Autodesk Fusion 360 part; units mm, degrees
sketch "Esquisse1" plane through (0, 0, 0) normal (0, 1, 0) x (1, 0, 0)
  arc A0 (59.719, 39.219) -> (44.719, 54.219) centre (44.719, 39.219) ccw construction
  line L0 (-39.219, -59.719) -> (44.719, -59.719) construction
  line L1 (-54.219, 39.219) -> (-54.219, -44.719) construction
  line L2 (-54.219, 54.219) -> (59.719, -59.719) construction
  line L3 (54.219, -12.5) -> (54.219, 12.5) construction
  arc A1 (44.719, -59.719) -> (59.719, -44.719) centre (44.719, -44.719) ccw construction
  arc A2 (-54.219, -44.719) -> (-39.219, -59.719) centre (-39.219, -44.719) ccw construction
  line L4 (44.719, 54.219) -> (-39.219, 54.219) construction
  line L5 (59.719, -44.719) -> (59.719, 39.219) construction
  arc A3 (-39.219, 54.219) -> (-54.219, 39.219) centre (-39.219, 39.219) ccw construction
  line L6 (-54.519, 39.219) -> (-54.519, -44.719)
  arc A4 (-54.519, -44.719) -> (-39.219, -60.019) centre (-39.219, -44.719) ccw
  line L7 (-39.219, -60.019) -> (44.719, -60.019)
  arc A5 (44.719, -60.019) -> (60.019, -44.719) centre (44.719, -44.719) ccw
  line L8 (60.019, -44.719) -> (60.019, 39.219)
  arc A6 (60.019, 39.219) -> (44.719, 54.519) centre (44.719, 39.219) ccw
  line L9 (44.719, 54.519) -> (-39.219, 54.519)
  arc A7 (-39.219, 54.519) -> (-54.519, 39.219) centre (-39.219, 39.219) ccw
  line L10 (-64.519, 39.219) -> (-64.519, -44.719)
  arc A8 (-64.519, -44.719) -> (-39.219, -70.019) centre (-39.219, -44.719) ccw
  line L11 (-39.219, -70.019) -> (44.719, -70.019)
  arc A9 (44.719, -70.019) -> (70.019, -44.719) centre (44.719, -44.719) ccw
  line L12 (70.019, -44.719) -> (70.019, 39.219)
  arc A10 (70.019, 39.219) -> (44.719, 64.519) centre (44.719, 39.219) ccw
  line L13 (44.719, 64.519) -> (-39.219, 64.519)
  arc A11 (-39.219, 64.519) -> (-64.519, 39.219) centre (-39.219, 39.219) ccw
  line L14 (-39.219, -65.019) -> (44.719, -65.019)
  arc A12 (44.719, -65.019) -> (65.019, -44.719) centre (44.719, -44.719) ccw
  line L15 (65.019, -44.719) -> (65.019, 39.219)
  arc A13 (65.019, 39.219) -> (44.719, 59.519) centre (44.719, 39.219) ccw
  line L16 (44.719, 59.519) -> (-39.219, 59.519)
  arc A14 (-39.219, 59.519) -> (-59.519, 39.219) centre (-39.219, 39.219) ccw
  line L17 (-59.519, 39.219) -> (-59.519, -44.719)
  arc A15 (-59.519, -44.719) -> (-39.219, -65.019) centre (-39.219, -44.719) ccw
  point P0 (54.219, 0)
  point P1 (54.219, 0)
  dimension "d2" = 15
  dimension "d3" = 15
  dimension "d4" = 113.9381
  dimension "d11" = 0.3
  dimension "d12" = 10
  dimension "d13" = 5
extrude "Extrusion1" add sketch "Esquisse1" along normal blind 153 contours L10 A8 L11 A9 L12 A10 L13 A11 | L14 A12 L15 A13 L16 A14 L17 A15
extrude "Extrusion2" cut sketch "Esquisse1" along normal blind 2 contours L14 A12 L15 A13 L16 A14 L17 A15
sketch "Esquisse2" plane through (0, 153, 0) normal (0, 1, 0) x (-1, 0, 0)
  arc A0 (39.219, -54.519) -> (54.519, -39.219) centre (39.219, -39.219) ccw
  line L0 (39.219, -54.519) -> (-44.719, -54.519)
  arc A1 (-60.019, -39.219) -> (-44.719, -54.519) centre (-44.719, -39.219) ccw
  line L1 (-60.019, -39.219) -> (-60.019, 44.719)
  arc A2 (-44.719, 60.019) -> (-60.019, 44.719) centre (-44.719, 44.719) ccw
  line L2 (-44.719, 60.019) -> (39.219, 60.019)
  arc A3 (54.519, 44.719) -> (39.219, 60.019) centre (39.219, 44.719) ccw
  line L3 (54.519, 44.719) -> (54.519, -39.219)
  arc A4 (39.219, -64.519) -> (64.519, -39.219) centre (39.219, -39.219) ccw
  line L4 (64.519, -39.219) -> (64.519, 44.719)
  arc A5 (64.519, 44.719) -> (39.219, 70.019) centre (39.219, 44.719) ccw
  line L5 (39.219, 70.019) -> (-44.719, 70.019)
  arc A6 (-44.719, 70.019) -> (-70.019, 44.719) centre (-44.719, 44.719) ccw
  line L6 (-70.019, 44.719) -> (-70.019, -39.219)
  arc A7 (-70.019, -39.219) -> (-44.719, -64.519) centre (-44.719, -39.219) ccw
  line L7 (-44.719, -64.519) -> (39.219, -64.519)
extrude "Extrusion3" add sketch "Esquisse2" along normal blind 10 contours A0 L0 A1 L1 A2 L2 A3 L3 | A4 L4 A5 L5 A6 L6 A7 L7
fillet "Congé1" radius 2 8 edges at (-54.519, 153, 2.75) (-50.0378, 153, -50.0378) (2.75, 153, -54.519) (55.5378, 153, -50.0378) (60.019, 153, 2.75) (55.5378, 153, 55.5378) (2.75, 153, 60.019) (-50.0378, 153, 55.5378)
fillet "Congé2" radius 1 8 edges at (-64.519, 163, 2.75) (-57.1088, 163, 62.6088) (2.75, 163, 70.019) (62.6088, 163, 62.6088) (70.019, 163, 2.75) (62.6088, 163, -57.1088) (2.75, 163, -64.519) (-57.1088, 163, -57.1088)
sketch "Esquisse3" plane through (-64.519, 0, 0) normal (-1, 0, 0) x (0, 0, 1)
  line L0 (44.719, 162) -> (-39.219, 162)
  line L1 (-39.219, 162) -> (-39.219, 0)
  line L2 (-39.219, 0) -> (44.719, 0)
  line L3 (44.719, 0) -> (44.719, 162)
  line L4 (-10.75, 49) -> (10.75, 49) construction
  line L5 (10.75, 49) -> (10.75, 0) construction
  line L6 (-10.75, 0) -> (-10.75, 49) construction
  circle A0 centre (-7.25, 45.5) radius 1.55
  circle A1 centre (7.25, 45.5) radius 1.55
  line L7 (-7.25, 45.5) -> (7.25, 45.5) construction
  line L8 (2.75, 162) -> (2.75, 132) construction
  line L9 (-17.25, 132) -> (22.75, 132) construction
  circle A2 centre (22.75, 132) radius 5.1
  circle A3 centre (-17.25, 132) radius 5.1
  line L10 (2.75, 132) -> (2.75, 97.36) construction
  circle A4 centre (2.75, 97.36) radius 5.1
  point P0 (2.75, 132)
  dimension "d24" = 49
  dimension "d25" = 21.5
  dimension "d26" = 3.1
  dimension "d27" = 3.1
  dimension "d28" = 14.5
  dimension "d29" = 3.5
  dimension "d30" = 3.5
  dimension "d31" = 30
  dimension "d32" = 40
  dimension "d33" = 34.64
  dimension "d34" = 10.2
  dimension "d35" = 10.2
  dimension "d36" = 10.2
extrude "Extrusion4" cut sketch "Esquisse3" against normal blind 2000 contours A0
extrude "Extrusion5" cut sketch "Esquisse3" against normal blind 2000 contours A1 | A2 | A3 | A4
scale "Echelle2" factor 1.075 about (44.719, 163, -63.519) bodies 1
equation "d4 = ( 430 mm - d2 * ( 2 * 3.141592 - 8 ) ) / 4"
equation "d33 = 0.866 * d32"
The model under review builds one solid part; all positions refer to its coordinate system, in mm. A direction names the side the tool comes from. Round coordinates to 2 decimals unless told otherwise and drop trailing zeros. Write each loop counter-clockwise with the first axis right and the second up, starting at its lowest first coordinate (ties: lowest second). Pieces come first, ordered by that corner, then holes. Notation, with made-up numbers: (15.25, 44) - (20.25, 44) arc R22 cw to (20.25, 62) - close; hole circle Ø5 at (19, 7.5). An arc over 180 degrees is marked (long way). One line per item, written item: value. Start each with the question number.
1. The part is to be moulded in two halves that separate along Y. For faces 1 (the face through (-67, 87, 7)), 2 (the face through (0, 152.25, 9)), 3 (the face through (-64.956, 73.631, -56.415)), say which applies: released by +Y, released by -Y, zero draft, split by the parting line, or undercut.
2. Consider section B-B on z = 7. State how many separate pieces and enclosed holes the cut face has, and give its area (3 significant figures).
3. Consider section C-C on x = 26.5. Write out the cut boundary in (y, z) (3 decimals), and give its area (3 significant figures).
4. Clearance check with flat-ended pins moving along their axes: P1, Ø10, axis at y = 29, z = -45, coming from the +X side; P2, Ø10, axis at x = -22, z = 9, coming from the -Y side. State where each tip first meets the part, or that it passes through.
5. Consider section A-A on y = 112.5. Write out the cut boundary in (x, z) (1 decimal), and give its area (3 significant figures).
6. To check wall thickness, follow L1, parallel to X at y = 136, z = -36; L2, parallel to Z at x = 16, y = 59.5; L3, parallel to Z at x = -21.5, y = 150.5. State the ranges of each line that lie inside material, in increasing order. Write a range as from..to.
7. Machinability: for faces 4 (the face through (-67.41, 135.11, 28.51)), 5 (the face through (59.979, -11.165, -52.996)), which of the approach directions +Z, -Z, +X, -X, +Y, -Y give a long, thin tool a straight path to every point of the face, cutting with its end or side? Answer none if there is none.
Checks:
1. face 1: undercut
1. face 2: released by -Y
1. face 3: zero draft
2. separate pieces: 3
2. enclosed holes: 0
2. area: 4,840 mm^2
3. outline: (-12.225, -64.594) - (161.925, -64.594) arc R1.075 ccw to (163, -63.519) - (163, 78.959) arc R1.075 ccw to (161.925, 80.034) - (-12.225, 80.034) - (-12.225, 74.659) - (-10.075, 74.659) - (-10.075, 69.284) - (150.1, 69.284) arc R2.15 cw to (152.25, 67.134) - (152.25, -51.694) arc R2.15 cw to (150.1, -53.844) - (-10.075, -53.844) - (-10.075, -59.219) - (-12.225, -59.219) - close
3. area: 5,070 mm^2
4. P1: stops at x = 71.79
4. P2: stops at y = 152.25
5. outline: (-72.7, -37.4) arc R27.2 ccw to (-45.5, -64.6) - (44.7, -64.6) arc R27.2 ccw to (71.9, -37.4) - (71.9, 52.8) arc R27.2 ccw to (44.7, 80) - (-45.5, 80) arc R27.2 ccw to (-72.7, 52.8) - close; hole (-62, -37.4) arc R16.4 ccw to (-45.5, -53.8) - (44.7, -53.8) arc R16.4 ccw to (61.2, -37.4) - (61.2, 52.8) arc R16.4 ccw to (44.7, 69.3) - (-45.5, 69.3) arc R16.4 ccw to (-62, 52.8) - close
5. area: 5,350 mm^2
6. L1: x = -72.71..-61.96, 61.17..71.92
6. L2: z = -64.59..-53.84, 69.28..80.03
6. L3: z = -64.59..-53.81, 69.25..80.03
7. face 4: +X, -X
7. face 5: -Y
